Autodesk Inventor part; units mm, degrees
ref_plane "YZ Plane" through (0, 0, 0) normal (1, 0, 0) x (0, 1, 0)
ref_plane "XZ Plane" through (0, 0, 0) normal (0, 1, 0) x (-1, 0, 0)
ref_plane "XY Plane" through (0, 0, 0) normal (0, 0, 1) x (1, 0, 0)
sketch "Sketch1" plane through (0, 0, 0) normal (0, 1, 0) x (-1, 0, 0)
  line L0 (15.4432, 14.405) -> (-15.4432, 14.405)
  line L1 (-15.4432, 14.405) -> (-15.4432, -14.405)
  line L2 (-15.4432, -14.405) -> (15.4432, -14.405)
  line L3 (15.4432, -14.405) -> (15.4432, 14.405)
  circle A0 centre (13.2432, -12.205) radius 1.5
  circle A1 centre (13.2432, 12.205) radius 1.5
  circle A2 centre (-13.2428, -12.205) radius 1.5
  circle A3 centre (-13.2428, 12.205) radius 1.5
  point P0 (0, 0)
  dimension "d0" = 30.8864
  dimension "d1" = 28.81
  dimension "d2" = 3
  dimension "d6" = 2.2
  dimension "d7" = 2.2
  dimension "d16" = 24.41
  dimension "d19" = 26.486
extrude "Extrusion1" add sketch "Sketch1" along normal blind 15
sketch "Sketch2" plane through (0, 0, 0) normal (0, -1, 0) x (1, 0, 0)
  circle A0 centre (13.2428, 12.205) radius 1.5
  circle A1 centre (13.2428, -12.205) radius 1.5
  circle A2 centre (-13.2432, 12.205) radius 1.5
  circle A3 centre (-13.2432, -12.205) radius 1.5
  line L0 (-15.4432, 14.405) -> (15.4432, 14.405)
  line L1 (-15.4432, -14.405) -> (-15.4432, 14.405)
  line L2 (15.4432, -14.405) -> (-15.4432, -14.405)
  line L3 (15.4432, 14.405) -> (15.4432, -14.405)
  circle A4 centre (13.2428, -12.205) radius 1.5
  line L4 (13.2428, -12.205) -> (-13.2432, 12.205)
  circle A5 centre (-13.2432, -12.205) radius 1.5
  line L5 (13.2428, 12.205) -> (-13.2432, -12.205)
  point P0 (0, 0)
sketch "Sketch3" plane through (0, 15, 0) normal (0, 1, 0) x (1, 0, 0)
  circle A0 centre (13.2428, -12.205) radius 1.5
  circle A1 centre (13.2428, 12.205) radius 1.5
  circle A2 centre (-13.2432, -12.205) radius 1.5
  circle A3 centre (-13.2432, 12.205) radius 1.5
  line L0 (-15.4432, -14.405) -> (15.4432, -14.405)
  line L1 (15.4432, -14.405) -> (15.4432, 14.405)
  line L2 (15.4432, 14.405) -> (-15.4432, 14.405)
  line L3 (-15.4432, 14.405) -> (-15.4432, -14.405)
  line L4 (23.1035, -2.0134) -> (-26.5318, -2.0134) construction
  line L5 (-26.5318, -2.0134) -> (-26.5318, 1.4328) construction
  line L6 (-26.5318, 1.4328) -> (23.1035, 1.4328) construction
  line L7 (23.1035, 1.4328) -> (23.1035, -2.0134) construction
  point P0 (0, 0)
properties part number "SoundDetectBaru"
For this review, take the finished solid that the model builds, in its own axes (mm). Round coordinates to 2 decimals unless told otherwise and drop trailing zeros. Loops run counter-clockwise (first coordinate to the right, second up) from the corner with the lowest first, then second, coordinate; pieces in that order, holes last.
(1) We need section A-A (z = -11.5). Give the boundary of the cut face in (x, y).
Returned:
outline: (-15.44, 0) - (-14.57, 0) - (-14.57, 15) - (-15.44, 15) - close; (-11.92, 0) - (11.92, 0) - (11.92, 15) - (-11.92, 15) - close; (14.57, 0) - (15.44, 0) - (15.44, 15) - (14.57, 15) - close
(2) We need section B-B (y = 8.5). Give the boundary of the cut face in (x, z) (3 decimals).
Returned:
outline: (-15.443, -14.405) - (15.443, -14.405) - (15.443, 14.405) - (-15.443, 14.405) - close; hole circle Ø3 at (-13.243, -12.205); hole circle Ø3 at (-13.243, 12.205); hole circle Ø3 at (13.243, -12.205); hole circle Ø3 at (13.243, 12.205)
(3) Mouldability with a two-part tool opening along X and no side actions: class faces 1 (the cylindrical face through (-14.63, 7.4, 12.78)), 2 (the flat face through (0, 7, -14.405)), 3 (the flat face through (-15.443, 7, 0)) as released by +X, released by -X, zero draft, split by the parting line, or undercut.
Returned:
face 1: undercut
face 2: zero draft
face 3: released by -X
(4) Wall thickness on line 1 along X through (y, z) = (14.5, -11.75); line 2 along Z through (x, y) = (14, 1.25) (3 decimals); line 3 along Z through (x, y) = (12, 6.25) (3 decimals): over which ranges is each line inside the solid? List them lowest first.
Returned:
line 1: x = -15.44 to -14.67, -11.81 to 11.81, 14.67 to 15.44
line 2: z = -14.405 to -13.5, -10.91 to 10.91, 13.5 to 14.405
line 3: z = -14.405 to -13.045, -11.365 to 11.365, 13.045 to 14.405
